The model under review builds one solid part; all positions refer to its coordinate system, in mm. A direction names the side the tool comes from. Round coordinates to 2 decimals unless told otherwise and drop trailing zeros. Order: outer loops, then holes, each group sorted by start corner. A loop starts at its lowest first (then second) coordinate and runs counter-clockwise, first axis right, second up. Notation, with made-up numbers: (-15, 61.25) -> (41, 61.25) arc R13 cw to (41, 86.25) -> close; hole circle Ø11 at (9, 79.5). An arc over 180 degrees is marked (long way). Use a Markdown table: item, result. Add a question column.
```python
from build123d import *

# Parameters (mm, degrees)
BOSS_EXTRUDE1_DEPTH   = 8.466666667
SKETCH2_R             = 16.885394085
SKETCH2_R_2           = 20.512287495
SKETCH2_R_3           = 19.572941721
CUT_EXTRUDE3_DEPTH    = 304.774506345
BOSS_EXTRUDE2_START   = 12.7
SKETCH2_4_R           = 20.695394085
SKETCH2_4_R_2         = 16.885394085
SKETCH2_4_R_3         = 24.322287495
SKETCH2_4_R_4         = 20.512287495
SKETCH2_4_R_5         = 23.382941721
SKETCH2_4_R_6         = 19.572941721
BOSS_EXTRUDE2_DEPTH   = 12.7
MIRROR3_START         = 33.866666667
MIRROR3_OUTLINE_R     = 19.572941721
MIRROR3_OUTLINE_R_2   = 20.512287495
MIRROR3_OUTLINE_R_3   = 16.885394085
MIRROR3_DEPTH         = 8.466666666
MIRROR3_START_2       = 21.166666667
MIRROR3_2_OUTLINE_R   = 23.382941721
MIRROR3_2_OUTLINE_R_2 = 19.572941721
MIRROR3_2_OUTLINE_R_3 = 24.322287495
MIRROR3_2_OUTLINE_R_4 = 20.512287495
MIRROR3_2_OUTLINE_R_5 = 20.695394085
MIRROR3_2_OUTLINE_R_6 = 16.885394085
MIRROR3_2_DEPTH       = 12.7


# Read off the part's stored shape, not the designer's step: Mirror3
with BuildPart() as part:
    # Sketch1 → Boss-Extrude1 (new body)
    with BuildSketch(Plane(origin=(0, 0, 0), x_dir=(1, 0, 0), z_dir=(0, 1, 0))):
        with BuildLine():
            Line((164.261221292, 12.021360676), (227.761221292, 12.021360676))
            ThreePointArc((227.761221292, 12.021360676), (219.55639394, -110.223196762), (127.314749355, -190.861463232))
            Line((127.314749355, -190.861463232), (6.974690834, -190.861455535))
            ThreePointArc((6.974690834, -190.861455535), (127.636363086, -121.995154476), (164.261221292, 12.021360676))
        make_face()
    extrude(amount=BOSS_EXTRUDE1_DEPTH)

    # Sketch2 → Cut-Extrude3 (cut, through all)
    with BuildSketch(Plane(origin=(0, 8.466666667, 0), x_dir=(1, 0, 0), z_dir=(0, 1, 0))):
        with Locations(Location((196.950964228, -18.851615567, 0), (0, 0, 270))):
            Circle(SKETCH2_R)
        with Locations(Location((189.259581589, -83.843798865, 0), (0, 0, 270))):
            Circle(SKETCH2_R_2)
        with Locations(Location((150.418099263, -143.836583448, 0), (0, 0, 270))):
            Circle(SKETCH2_R_3)
    extrude(amount=-CUT_EXTRUDE3_DEPTH, mode=Mode.SUBTRACT)

    # Sketch2_4 → Boss-Extrude2 (add)
    # profile 1 of 3: a face of its own
    with BuildSketch(Plane(origin=(0, 8.466666667, 0), x_dir=(1, 0, 0), z_dir=(0, 1, 0)).offset(BOSS_EXTRUDE2_START)):
        with Locations(Location((196.950964228, -18.851615567, 0), (0, 0, 90))):
            Circle(SKETCH2_4_R)
        with Locations(Location((196.950964228, -18.851615567, 0), (0, 0, 270))):
            Circle(SKETCH2_4_R_2, mode=Mode.SUBTRACT)
    # profile 2 of 3: a face of its own
    with BuildSketch(Plane(origin=(0, 8.466666667, 0), x_dir=(1, 0, 0), z_dir=(0, 1, 0)).offset(BOSS_EXTRUDE2_START)):
        with Locations(Location((189.259581589, -83.843798865, 0), (0, 0, 90))):
            Circle(SKETCH2_4_R_3)
        with Locations(Location((189.259581589, -83.843798865, 0), (0, 0, 270))):
            Circle(SKETCH2_4_R_4, mode=Mode.SUBTRACT)
    # profile 3 of 3: a face of its own
    with BuildSketch(Plane(origin=(0, 8.466666667, 0), x_dir=(1, 0, 0), z_dir=(0, 1, 0)).offset(BOSS_EXTRUDE2_START)):
        with Locations(Location((150.418099263, -143.836583448, 0), (0, 0, 90))):
            Circle(SKETCH2_4_R_5)
        with Locations(Location((150.418099263, -143.836583448, 0), (0, 0, 270))):
            Circle(SKETCH2_4_R_6, mode=Mode.SUBTRACT)
    extrude(amount=-BOSS_EXTRUDE2_DEPTH)



with BuildPart() as body_2:
    # Mirror3 outline → Mirror3 (new body)
    with BuildSketch(Plane(origin=(0, 0, 0), x_dir=(1, 0, 0), z_dir=(0, 1, 0)).offset(MIRROR3_START)):
        with BuildLine():
            ThreePointArc((164.261221292, 12.021360676), (127.636363086, -121.995154476), (6.974690834, -190.861455535))
            Line((6.974690834, -190.861455535), (127.314749355, -190.861463232))
            ThreePointArc((127.314749355, -190.861463232), (219.55639394, -110.223196762), (227.761221292, 12.021360676))
            Line((227.761221292, 12.021360676), (164.261221292, 12.021360676))
        make_face()
        with Locations((150.418099263, -143.836583448)):
            Circle(MIRROR3_OUTLINE_R, mode=Mode.SUBTRACT)
        with Locations((189.259581589, -83.843798865)):
            Circle(MIRROR3_OUTLINE_R_2, mode=Mode.SUBTRACT)
        with Locations((196.950964228, -18.851615567)):
            Circle(MIRROR3_OUTLINE_R_3, mode=Mode.SUBTRACT)
    extrude(amount=MIRROR3_DEPTH)


with BuildPart() as part_1:
    add(part.part)

    add(body_2.part)  # Mirror3 2 merges body 2
    # Mirror3 2 outline → Mirror3 2 (add)
    # profile 1 of 3: a face of its own
    with BuildSketch(Plane(origin=(0, 0, 0), x_dir=(1, 0, 0), z_dir=(0, 1, 0)).offset(MIRROR3_START_2)):
        with Locations((150.418099263, -143.836583448)):
            Circle(MIRROR3_2_OUTLINE_R)
        with Locations((150.418099263, -143.836583448)):
            Circle(MIRROR3_2_OUTLINE_R_2, mode=Mode.SUBTRACT)
    # profile 2 of 3: a face of its own
    with BuildSketch(Plane(origin=(0, 0, 0), x_dir=(1, 0, 0), z_dir=(0, 1, 0)).offset(MIRROR3_START_2)):
        with Locations((189.259581589, -83.843798865)):
            Circle(MIRROR3_2_OUTLINE_R_3)
        with Locations((189.259581589, -83.843798865)):
            Circle(MIRROR3_2_OUTLINE_R_4, mode=Mode.SUBTRACT)
    # profile 3 of 3: a face of its own
    with BuildSketch(Plane(origin=(0, 0, 0), x_dir=(1, 0, 0), z_dir=(0, 1, 0)).offset(MIRROR3_START_2)):
        with Locations((196.950964228, -18.851615567)):
            Circle(MIRROR3_2_OUTLINE_R_5)
        with Locations((196.950964228, -18.851615567)):
            Circle(MIRROR3_2_OUTLINE_R_6, mode=Mode.SUBTRACT)
    extrude(amount=MIRROR3_2_DEPTH)


solid = part_1.part
```
Q1. Mouldability with a two-part tool opening along Y and no side actions: class faces 3 (the cylindrical face through (216.16, 23.81, 11.15)), 4 (the flat face through (163, 42.333, 96)), 5 (the flat face through (196, 38, -12.021)) as pulls with the +Y half, pulls with the -Y half, needs draft (parallel to the pull), parting line crosses it, or undercut.
Q2. Insertion check: pin 1 (2 mm diameter, centred on y = 32.5, z = 144, fed in from +X); pin 2 (4 mm diameter, centred on x = 62, y = 38, fed in from -Z); pin 3 (10 mm diameter, centred on x = 44, y = 30.5, fed in from -Z). Each pin has a flat end and moves straight along its axis. Give the tip position at first contact, or say it passes through.
Q3. Wall thickness on line 1 (Z direction, x = 208, y = 34); line 2 (Y direction, x = 109, z = 169); line 3 (X direction, y = 4, z = 69.5): over which ranges is each line inside the solid? List them lowest first. Write a range as [from, to].
Q4. Add section A-A (x = 67). Write out the cut boundary in (y, z), then the cut area to 3 significant figures.
Q5. Add section B-B (z = 11.5). Write out the cut boundary in (x, y).
Q6. Machinability: for faces 1 (the cylindrical face through (172.12, 23.81, 135.13)), 2 (the cylindrical face through (218.767, 38.041, 111.796)), which of the approach directions +Z, -Z, +X, -X, +Y, -Y give a long, thin tool a straight path to every point of the face, cutting with its end or side? Answer none if there is none.
Q7. Add section C-C (y = 38). Write out the cut boundary in (x, z).
Q8. Add section D-D (x = 124.5). Write out the cut boundary in (y, z), then the cut area to 3 significant figures.
Report:
| question | item | result |
|---|---|---|
| 1 | face 3 | undercut |
| 1 | face 4 | pulls with the +Y half |
| 1 | face 5 | needs draft |
| 2 | pin 1 | stops at x = 173.8 |
| 2 | pin 2 | stops at z = 173.81 |
| 2 | pin 3 | stops at z = 180.82 |
| 3 | line 1 | z = [-12.02, 6.08], [31.62, 75.5], [92.18, 129.9] |
| 3 | line 2 | y = [0, 8.47], [33.87, 42.33] |
| 3 | line 3 | x = [155.94, 174.6], [203.92, 233.28] |
| 4 | outline | (0, 172.3) -> (8.47, 172.3) -> (8.47, 190.86) -> (0, 190.86) -> close; (33.87, 172.3) -> (42.33, 172.3) -> (42.33, 190.86) -> (33.87, 190.86) -> close |
| 4 | area | 314 mm² |
| 5 | outline | (165.7, 0) -> (181.75, 0) -> (181.75, 42.33) -> (165.7, 42.33) -> (165.7, 33.87) -> (177.61, 33.87) -> (177.61, 8.47) -> (165.7, 8.47) -> close; (212.15, 0) -> (233.76, 0) -> (233.76, 8.47) -> (216.3, 8.47) -> (216.3, 33.87) -> (233.76, 33.87) -> (233.76, 42.33) -> (212.15, 42.33) -> close |
| 6 | face 1 | none |
| 6 | face 2 | +X, +Y, -Y |
| 7 | outline | (6.97, 190.86) arc R181.52 cw to (164.26, -12.02) -> (227.76, -12.02) arc R160.08 ccw to (127.31, 190.86) -> close; hole circle Ø39.15 at (150.42, 143.84); hole circle Ø41.02 at (189.26, 83.84); hole circle Ø33.77 at (196.95, 18.85) |
| 8 | outline | (0, 125.93) -> (8.47, 125.93) -> (8.47, 190.86) -> (0, 190.86) -> close; (33.87, 125.93) -> (42.33, 125.93) -> (42.33, 190.86) -> (33.87, 190.86) -> close |
| 8 | area | 1,100 mm² |
